Autodesk Inventor part; units mm, degrees
ref_plane "YZ Plane" through (0, 0, 0) normal (1, 0, 0) x (0, 1, 0)
ref_plane "XZ Plane" through (0, 0, 0) normal (0, 1, 0) x (-1, 0, 0)
ref_plane "XY Plane" through (0, 0, 0) normal (0, 0, 1) x (1, 0, 0)
sketch "Sketch4" plane through (0, 0, 0) normal (1, 0, 0) x (0, 1, 0)
  circle A0 centre (0, 0) radius 2.75
  circle A1 centre (0, 0) radius 5
  dimension "d19" = 5.5
  dimension "d20" = 10
extrude "Extrusion2" add sketch "Sketch4" along normal blind 10 contours A0 | A1
sketch "Sketch5" plane through (0, 0, 0) normal (-1, 0, 0) x (0, 0, 1)
  circle A0 centre (0, 0) radius 2.75
  dimension "d23" = 5.5
hole "Hole3" at (0, 0, 0) direction (1, 0, 0) diameter 5.5 depth 5
sketch "Sketch6" plane through (10, 0, 0) normal (1, 0, 0) x (0, 0, -1)
  circle A0 centre (0, 0) radius 3.5
  dimension "d31" = 7
extrude "Extrusion3" add sketch "Sketch6" along normal blind 10
sketch "Sketch7" plane through (20, 0, 0) normal (1, 0, 0) x (0, 0, -1)
  circle A0 centre (0, 0) radius 3
  dimension "d34" = 6
hole "Hole4" at (20, 0, 0) direction (-1, 0, 0) diameter 3.5 depth 5
properties part number "acople"
Source: CAD feature listing. Evaluate the final solid. Frame: model axes, mm. A direction names the side the tool comes from. Coordinates: 2 decimals unless noted, no trailing zeros. Loops run counter-clockwise (first coordinate to the right, second up) from the corner with the lowest first, then second, coordinate; pieces in that order, holes last. Notation, with made-up numbers: (-20.75, 41.5) -> (-15.75, 41.5) arc R16 cw to (-15.75, 46.5) -> close; hole circle Ø2 at (14, -0.75). An arc over 180 degrees is marked (long way). One line per item, written item: value. Start each with the question number.
Q1. Section query C-C, the plane x = 4.5. Return the cut outline in (y, z), and give its area (3 significant figures).
Q2. Line query: line 1 along Z through (x, y) = (3.1, 0); line 2 along X through (y, z) = (-3.75, -0.25); line 3 along Y through (x, z) = (18, 0). Output: solid intervals per line, ascending.
Q3. Mould query, pull axis Y, two halves, no side actions, for faces 1 (the face through (10, 2.2, -3.3)), 2 (the face through (4.93, -1.08, 4.88)), 3 (the face through (17.465, 0.67, -1.617)). Classes: pulls with the +Y half, pulls with the -Y half, needs draft (parallel to the pull), parting line crosses it, or undercut.
Q4. Contact query for flat-ended pins moving along their axis: P1, Ø1.5, axis at y = -1, z = 0.5, coming from the +X side; P2, Ø1.6, axis at y = -0.5, z = -1, coming from the -X side; P3, Ø2, axis at y = -3, z = 4, coming from the +X side; P4, Ø3, axis at x = 2, y = -3, coming from the -Z side. Output: stop coordinate, or through.
Q5. Section query D-D, the plane x = 14.5. Return the cut outline in (y, z).
Q6. Section query A-A, the plane y = 0. Return the cut outline in (x, z).
Q7. Set-up query: faces 4 (the face through (15, 0, 0)), 5 (the face through (5, 0, 0)), 6 (the face through (20, -1, 2)). Return all of +Z, -Z, +X, -X, +Y, -Y with unobstructed straight access to the full face (end or side cutting, diameter ignored); none if empty.
Results:
1. outline: circle Ø10 at (0, 0); hole circle Ø5.5 at (0, 0)
1. area: 54.8 mm^2
2. line 1: -5 to -2.75, 2.75 to 5
2. line 2: 0 to 10
2. line 3: -3.5 to -1.75, 1.75 to 3.5
3. face 1: needs draft
3. face 2: parting line crosses it
3. face 3: undercut
4. P1: x = 20
4. P2: x = 5
4. P3: x = 10
4. P4: z = -4.77
5. outline: circle Ø7 at (0, 0)
6. outline: (0, -5) -> (10, -5) -> (10, -3.5) -> (20, -3.5) -> (20, -1.75) -> (15, -1.75) -> (15, 1.75) -> (20, 1.75) -> (20, 3.5) -> (10, 3.5) -> (10, 5) -> (0, 5) -> (0, 2.75) -> (5, 2.75) -> (5, -2.75) -> (0, -2.75) -> close
7. face 4: +X
7. face 5: -X
7. face 6: +Z, -Z, +X, +Y, -Y
